```python
from build123d import *

# Parameters (mm, degrees)
F0_W     = 1200
F0_H     = 340
F1_DEPTH = 600
F3_DEPTH = 150
F4_W     = 400
F4_H     = 120
F5_DEPTH = 600.001
F7_DEPTH = 150
F8_R     = 110
F9_DEPTH = 490.001


# Not quite as in the source:
# - a feature names something its author has since deleted; it is built from what else it names


with BuildPart() as f1:
    # F0 (on Front) → F1 (new body)
    with BuildSketch(Plane.XZ):
        Rectangle(F0_W, F0_H)
    extrude(amount=F1_DEPTH)

    # F2 (on face) → F3 (cut)
    with BuildSketch(Plane.XY.offset(170)):
        with BuildLine():
            Line((-600, -150), (-600, -450))
            ThreePointArc((-600, -450), (-450, -300), (-600, -150))
        make_face()
        with BuildLine():
            ThreePointArc((600, -150), (450, -300), (600, -450))
            Line((600, -450), (600, -150))
        make_face()
    extrude(amount=-F3_DEPTH, mode=Mode.SUBTRACT)

    # F4 (on face) → F5 (cut, through all)
    with BuildSketch(Plane(origin=(0, 0, 0), x_dir=(-1, 0, 0), z_dir=(0, 1, 0))):
        with Locations((0, -110)):
            Rectangle(F4_W, F4_H)
    extrude(amount=-F5_DEPTH, mode=Mode.SUBTRACT)

    # F6 (on face) → F7 (join)
    with BuildSketch(Plane.XY.offset(170)):
        with BuildLine():
            Line((230, -100), (-230, -100))
            ThreePointArc((-230, -100), (-314.8528137424, -135.1471862576), (-350, -220))
            Line((-350, -220), (-350, -380))
            ThreePointArc((-350, -380), (-314.8528137424, -464.8528137424), (-230, -500))
            Line((-230, -500), (230, -500))
            ThreePointArc((230, -500), (314.8528137424, -464.8528137424), (350, -380))
            Line((350, -380), (350, -220))
            ThreePointArc((350, -220), (314.8528137424, -135.1471862576), (230, -100))
        make_face()
    extrude(amount=F7_DEPTH)

    # F8 (on face) → F9 (cut, through all)
    with BuildSketch(Plane.XY.offset(320)):
        with Locations((0, -300)):
            Circle(F8_R)
    extrude(amount=-F9_DEPTH, mode=Mode.SUBTRACT)


solid = f1.part
```
Input: part model. Units: mm. Frame: model coordinates. A direction names the side the tool comes from. Coordinates: 2 decimals unless noted, no trailing zeros. Loops run counter-clockwise (first coordinate to the right, second up) from the corner with the lowest first, then second, coordinate; pieces in that order, holes last. Notation, with made-up numbers: M -35.75,-8.75 L -25.75,-8.75 A21 cw -25.75,15.25 Z; hole C 21,16 d11. An arc over 180 degrees is marked long. Use a Markdown table: item, result. Add a question column.
1) Section B-B, the plane y = -300. Return the cut outline in (x, z).
2) Section C-C, the plane x = 0. Return the cut outline in (y, z).
3) Section A-A, the plane z = -127.5. Return the cut outline in (x, y), plus the area to 3 significant figures.
4) Line query: L1, parallel to Y at x = 0, z = 108.5; L2, parallel to X at y = -65, z = -131.5; L3, parallel to X at y = -358.5, z = 117. Output: solid intervals per line, ascending. Write a range as from..to.
5) Draft query along X for faces 1 (the flat face through (200, -296, -111)), 2 (the cylindrical face through (313.915, -465.781, 243.95)), 3 (the flat face through (-350, -299, 244)). Return one class per face: +X half, -X half, draft (parallel to the pull), parting line (faces both ways), or undercut.
6) Pin query (flat end, axial travel): P1, Ø1.5, axis at y = -345.5, z = 211.5, coming from the +X side; P2, Ø6, axis at x = -242.5, z = 221.5, coming from the +Y side. Return the tip coordinate at first contact, or that it passes through.
7) Set-up query: faces 4 (the flat face through (92, -229, -50)), 5 (the cylindrical face through (315.781, -136.085, 243.95)), 6 (the cylindrical face through (450.036, -296.702, 96.05)), 7 (the flat face through (3, -100, 244)). Return all of +Z, -Z, +X, -X, +Y, -Y with unobstructed straight access to the full face (end or side cutting, diameter ignored); none if empty.
8) Section D-D, the plane z = 85. Return the cut outline in (x, y), plus the area to 3 significant figures.
Answer below:
| question | item | result |
|---|---|---|
| 1 | outline | M -600,-170 L -200,-170 L -200,-50 L -110,-50 L -110,320 L -350,320 L -350,170 L -450,170 L -450,20 L -600,20 Z; M 110,-50 L 200,-50 L 200,-170 L 600,-170 L 600,20 L 450,20 L 450,170 L 350,170 L 350,320 L 110,320 Z |
| 2 | outline | M -600,-50 L -410,-50 L -410,320 L -500,320 L -500,170 L -600,170 Z; M -190,-50 L 0,-50 L 0,170 L -100,170 L -100,320 L -190,320 Z |
| 3 | outline | M -600,-600 L -200,-600 L -200,0 L -600,0 Z; M 200,-600 L 600,-600 L 600,0 L 200,0 Z |
| 3 | area | 480,000 mm2 |
| 4 | L1 | -600..-410, -190..0 |
| 4 | L2 | -600..-200, 200..600 |
| 4 | L3 | -461.88..-93.15, 93.15..461.88 |
| 5 | face 1 | undercut |
| 5 | face 2 | +X half |
| 5 | face 3 | -X half |
| 6 | P1 | x = 350 |
| 6 | P2 | y = -100.38 |
| 7 | face 4 | -Z, +Y, -Y |
| 7 | face 5 | +Z, +X, +Y |
| 7 | face 6 | +Z, +X |
| 7 | face 7 | +Z, +X, -X, +Y |
| 8 | outline | M -600,-600 L 600,-600 L 600,-450 A150 cw 600,-150 L 600,0 L -600,0 L -600,-150 A150 cw -600,-450 Z; hole C 0,-300 d220 |
| 8 | area | 611,000 mm2 |
